Solid Edge part; units mm, degrees
sketch "Sketch1" plane through (0, 0, 0) normal (0, -1, 0) x (1, 0, 0)
  line L0 (-395.3177, -45.9234) -> (-95.3177, -45.9234)
  line L1 (-95.3177, -45.9234) -> (-95.3177, 254.0766)
  line L2 (-95.3177, 254.0766) -> (-395.3177, 254.0766)
  line L3 (-395.3177, 254.0766) -> (-395.3177, -45.9234)
  dimension "D1" = 395.3177
  dimension "D2" = 95.3177
extrude "Protrusion1" add sketch "Sketch1" against normal blind 10
sketch "Sketch2" plane through (-145.3177, 0, 4.0766) normal (0, -1, 0) x (1, 0, 0)
  circle A0 centre (-30, 182) radius 6.5
  circle A1 centre (-182, 30) radius 6.5
  circle A2 centre (-30, 30) radius 6.5
  circle A3 centre (-182, 182) radius 6.5
extrude "Cutout1" cut sketch "Sketch2" along normal through all and the other way through all
sketch "Sketch3" plane through (-245.3177, 10, 104.0766) normal (0, 1, 0) x (1, 0, 0)
  circle A0 centre (-7, -7) radius 60.87
  line L0 (150, 150) -> (150, 90)
  line L1 (150, 90) -> (90, 90)
  line L2 (90, 90) -> (90, 150)
  line L3 (90, 150) -> (150, 150)
  dimension "D1" = 90
  dimension "D2" = 150
  dimension "D3" = 7
extrude "Cutout2" cut sketch "Sketch3" against normal through all
sketch "Sketch4" plane through (-245.3177, 0, 104.0766) normal (0, -1, 0) x (0, 0, -1)
  line L0 (-150, -60) -> (-60, -150)
  line L1 (-60, -150) -> (-150, -150)
  line L2 (-150, -150) -> (-150, -60)
  dimension "D1" = 150
  dimension "D2" = 60
extrude "Cutout3" cut sketch "Sketch4" against normal through all
Part model, mm, in its own coordinate system. A direction names the side the tool comes from. Coordinates: 2 decimals unless noted, no trailing zeros. Order: outer loops, then holes, each group sorted by start corner. A loop starts at its lowest first (then second) coordinate and runs counter-clockwise, first axis right, second up.
(1) Tool access for faces 4 (the face through (-199, 5, 254.077)), 5 (the face through (-155.318, 5, -16)): list every direction of +Z, -Z, +X, -X, +Y, -Y with a clear straight run to the whole face (end or side of a thin tool).
Check sheet entries:
face 4: +Z, +X, -X, +Y, -Y
face 5: -Z, +X, +Y, -Y
(2) Slice it at C-C, the plane y = 4.25. Write the cut outline in (x, z).
Check sheet entries:
outline: (-395.32, -45.92) - (-155.32, -45.92) - (-155.32, 14.08) - (-95.32, 14.08) - (-95.32, 254.08) - (-305.32, 254.08) - (-395.32, 164.08) - close; hole circle Ø13 at (-327.32, 34.08); hole circle Ø13 at (-327.32, 186.08); hole circle Ø121.74 at (-252.32, 111.08); hole circle Ø13 at (-175.32, 34.08); hole circle Ø13 at (-175.32, 186.08)
(3) Slice it at D-D, the plane z = -7.5. Write the cut outline in (x, y), and give its area (3 significant figures).
Check sheet entries:
outline: (-395.32, 0) - (-155.32, 0) - (-155.32, 10) - (-395.32, 10) - close
area: 2,400 mm2
(4) Probe L1, parallel to Z at x = -177, y = 3.5; L2, parallel to Z at x = -328.5, y = 3.5; L3, parallel to X at y = 7.75, z = 112. List the from-to ranges inside material, lowest first.
Check sheet entries:
L1: z = -45.92 to 27.8, 40.36 to 179.8, 192.36 to 254.08
L2: z = -45.92 to 27.69, 40.47 to 179.69, 192.47 to 230.89
L3: x = -395.32 to -313.18, -191.45 to -95.32
(5) Slice it at B-B, the plane x = -271. Write the cut outline in (y, z), and give its area (3 significant figures).
Check sheet entries:
outline: (0, -45.92) - (10, -45.92) - (10, 53.14) - (0, 53.14) - close; (0, 169.01) - (10, 169.01) - (10, 254.08) - (0, 254.08) - close
area: 1,840 mm2
(6) Slice it at A-A, the plane z = 158.5. Write the cut outline in (x, y), and give its area (3 significant figures).
Check sheet entries:
outline: (-395.32, 0) - (-290.48, 0) - (-290.48, 10) - (-395.32, 10) - close; (-214.16, 0) - (-95.32, 0) - (-95.32, 10) - (-214.16, 10) - close
area: 2,240 mm2
(7) Pin check, flat tips, straight feed: pin 1 Ø17 at (x, z) = (-175.32, 186.08) entering from +Y; pin 2 Ø1 at (y, z) = (4, 169.5) entering from -X; pin 3 Ø4 at (x, y) = (-360, 7) entering from +Z; pin 4 Ø3 at (x, y) = (-140, 7.5) entering from -Z. Stop position of each tip, or through.
Check sheet entries:
pin 1: stops at y = 10
pin 2: stops at x = -390.39
pin 3: stops at z = 201.39
pin 4: stops at z = 14.08
(8) Pull direction Z, two halves, no side cores. Call faces 1 (the face through (-277, 5, -45.923)), 2 (the face through (-243, 10, 173)), 3 (the face through (-169.12, 4.93, 36.03)): pulls with the +Z half, pulls with the -Z half, needs draft (parallel to the pull), parting line crosses it, or undercut.
Check sheet entries:
face 1: pulls with the -Z half
face 2: needs draft
face 3: undercut
